from build123d import *

# Parameters (mm, degrees)
SKETCH1_R             = 50.8
SKETCH1_R_2           = 15
BOSS_EXTRUDE1_DEPTH   = 6.35
CIRPATTERN1_COUNT     = 8
SKETCH5_R             = 41.25
CUT_EXTRUDE1_DEPTH    = 3.175
CHAMFER1_SIZE         = 0.7874
F_8_32_TAPPED_HOLE1_D = 3.4544
CIRPATTERN2_COUNT     = 6
BOSS_EXTRUDE3_START   = -6.35
BOSS_EXTRUDE3_DEPTH   = 6.35
FILLET2_R             = 6.35


with BuildPart() as part:
    # Sketch1 → Boss-Extrude1 (new body)
    with BuildSketch(Plane.XY):
        Circle(SKETCH1_R)
        Circle(SKETCH1_R_2, mode=Mode.SUBTRACT)
    extrude(amount=BOSS_EXTRUDE1_DEPTH)

    # Sketch4 → M4 Clearance Hole1 (revolve, cut)
    with BuildSketch(Plane(origin=(0, 21.249999918, 6.35), x_dir=(0, -1, 0), z_dir=(1, 0, 0))):
        Polygon((0, 0), (0, 26.751936393), (2.25, 25.4), (2.25, 0), align=None)
    m4_clearance_hole1 = revolve(axis=Axis((0, 21.249999918, 12.7), (0, 0, -1)), mode=Mode.SUBTRACT)

    # CirPattern1: M4 Clearance Hole1 ×8 about axis
    cirpattern1_axis = Axis((0, 0, 0), (0, 0, 1))
    for i in range(1, CIRPATTERN1_COUNT):
        add(m4_clearance_hole1.rotate(cirpattern1_axis, i * 360 / CIRPATTERN1_COUNT), mode=Mode.SUBTRACT)

    # Sketch5 → Cut-Extrude1 (cut)
    with BuildSketch(Plane(origin=(0, 0, 0), x_dir=(-1, 0, 0), z_dir=(0, 0, -1))):
        Circle(SKETCH5_R)
    extrude(amount=-CUT_EXTRUDE1_DEPTH, mode=Mode.SUBTRACT)

    # Chamfer1
    chamfer1_edges = [part.edges().sort_by_distance(p)[0] for p in [
        (41.25, 0, 0),
    ]]
    chamfer(chamfer1_edges, length=CHAMFER1_SIZE)

    # #8-32 Tapped Hole1 (through all)
    with Locations(Plane.XY.offset(6.35)):
        with Locations((0, 44.45)):
            f_8_32_tapped_hole1 = Hole(F_8_32_TAPPED_HOLE1_D / 2)

    # CirPattern2: #8-32 Tapped Hole1 ×6 about axis
    cirpattern2_axis = Axis((0, 0, 0), (0, 0, 1))
    for i in range(1, CIRPATTERN2_COUNT):
        add(f_8_32_tapped_hole1.rotate(cirpattern2_axis, i * 360 / CIRPATTERN2_COUNT), mode=Mode.SUBTRACT)

    # Sketch10 → Boss-Extrude3 (add)
    with BuildSketch(Plane.XY.offset(6.35).offset(BOSS_EXTRUDE3_START)):
        with BuildLine():
            ThreePointArc((5.073646026, 50.546), (0, 55.88), (-5.073646026, 50.546))
            ThreePointArc((-5.073646026, 50.546), (0, 50.8), (5.073646026, 50.546))
        make_face()
    extrude(amount=BOSS_EXTRUDE3_DEPTH)

    # Fillet2
    fillet2_edges = [part.edges().sort_by_distance(p)[0] for p in [
        (5.073646026, 50.546, 3.175),
        (-5.073646026, 50.546, 3.175),
    ]]
    fillet(fillet2_edges, radius=FILLET2_R)


solid = part.part
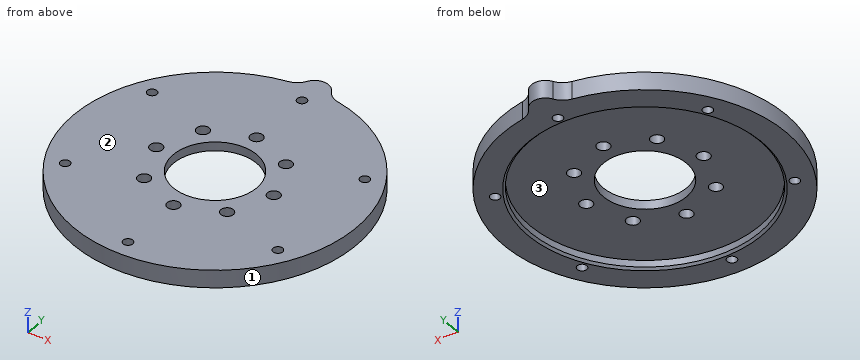
The model under review builds one solid part; all positions refer to its coordinate system, in mm. Face numbers are marked on the shaded views. Give positions to 0.01 mm unless a question says otherwise; leave off trailing zeros. Write each loop counter-clockwise with the first axis right and the second up, starting at its lowest first coordinate (ties: lowest second). Pieces come first, ordered by that corner, then holes.
1. Add section B-B, the plane y = -44.45. Write out the cut boundary in (x, z), plus the area to 3 significant figures.
2. Add section C-C, the plane z = 4.5. Count the separate pieces of the cut face and the enclosed holes in it, plus the area to 3 significant figures.
3. For P1, Ø3.5, axis at x = -15.03, y = 15.03, coming from the +Z side; P2, Ø2, axis at x = -35, z = 4, coming from the +Y side; P3, Ø3, axis at x = 34.5, z = 5, coming from the -Y side; P4, Ø5, axis at x = 0, y = -21.25, coming from the -Z side (3 decimals), all flat-tipped, find the tip position at first contact; note any pin that passes through.
4. Wall thickness on L1, parallel to Y at x = 0, z = 5.65; L2, parallel to Y at x = 0, z = 2.75; L3, parallel to Y at x = 17, z = 4.5: over which ranges is each line inside the solid? List them lowest first.
5. Add section D-D, the plane x = 44.5. Write out the cut boundary in (y, z).
6. Draft analysis for pull direction Y (two halves, no side actions). For the marked faces 1, 2 and 3, state which applies: +Y half, -Y half, draft (parallel to the pull), parting line (faces both ways), or undercut.
7. Add section A-A, the plane y = 0. Write out the cut boundary in (x, z) (3 decimals).
Worked answers:
1. outline: (-24.59, 0) - (-1.73, 0) - (-1.73, 6.35) - (-24.59, 6.35) - close; (1.73, 0) - (24.59, 0) - (24.59, 6.35) - (1.73, 6.35) - close
1. area: 290 mm2
2. separate pieces: 1
2. enclosed holes: 15
2. area: 7,260 mm2
3. P1: passes through
3. P2: stops at y = 37.74
3. P3: stops at y = -38.62
3. P4: stops at z = 3.175
4. L1: y = -50.8 to -46.18, -42.72 to -23.5, -19 to -15, 15 to 19, 23.5 to 42.72, 46.18 to 55.88
4. L2: y = -50.8 to -46.18, -42.72 to -41.25, 41.25 to 42.72, 46.18 to 55.88
4. L3: y = -47.87 to -16.11, -13.95 to 13.95, 16.11 to 47.87
5. outline: (-24.5, 0) - (24.5, 0) - (24.5, 6.35) - (-24.5, 6.35) - close
6. face 1: parting line
6. face 2: draft
6. face 3: undercut
7. outline: (-50.8, 0) - (-42.037, 0) - (-41.25, 0.787) - (-41.25, 3.175) - (-23.5, 3.175) - (-23.5, 6.35) - (-50.8, 6.35) - close; (-19, 3.175) - (-15, 3.175) - (-15, 6.35) - (-19, 6.35) - close; (15, 3.175) - (19, 3.175) - (19, 6.35) - (15, 6.35) - close; (23.5, 3.175) - (41.25, 3.175) - (41.25, 0.787) - (42.037, 0) - (50.8, 0) - (50.8, 6.35) - (23.5, 6.35) - close
